Can you work these out from the model? Positions are in its coordinate system, mm. A direction names the side the tool comes from. Round coordinates to 2 decimals unless told otherwise and drop trailing zeros. Order: outer loops, then holes, each group sorted by start corner. A loop starts at its lowest first (then second) coordinate and runs counter-clockwise, first axis right, second up. Notation, with made-up numbers: (27, -17.5) -> (68, -17.5) arc R18 ccw to (68, 7.5) -> close; hole circle Ø4 at (41, -7). An arc over 180 degrees is marked (long way). Use a Markdown table: item, result. Add a question column.
Q1. I need wall thicknesses on line 1 along X through (y, z) = (5.5, 2.85); line 2 along Y through (x, z) = (10, 1.5); line 3 along Y through (x, z) = (-10, 1.6). Which ranges of each line are inside material? Lowest first, please. Write a range as [from, to].
Q2. If we section it at D-D on z = 3.2: Give the number of separate pieces and of enclosed holes in the cut face, plus the area to 3 significant figures.
Q3. If we section it at A-A on x = 0: List the corners of the cut face in (y, z) for me, plus the area to 3 significant figures.
Q4. We'd pull the mould along X, two halves only. Please class faces 1 (the face through (-25.295, -5, 2)), 2 (the face through (0, 45, 2)), 3 (the face through (-27.14, 44.1, 2.03)), 4 (the face through (28, 8, 2)): +X half, -X half, draft (parallel to the pull), parting line (faces both ways), or undercut.
Q5. If we section it at B-B on y = 14.5: List the corners of the cut face in (x, z) for me.
Q6. For faces 5 (the face through (-10.85, 21.08, 2.03)), 6 (the face through (0, 1, 4)), which set-ups out of +Z, -Z, +X, -X, +Y, -Y let a thin tool reach every point of the face, with its end or its side?
Q7. I'm going to push flat-ended pins straight in: pin 1 Ø1.2 at (x, z) = (-18, 1.5) entering from -Y; pin 2 Ø2 at (y, z) = (-27, 3.5) entering from -X (3 decimals); pin 3 Ø2.5 at (x, y) = (-13.44, -3.56) entering from +Z. Where does each tip first touch, or does it pass through?
Q8. If we section it at C-C on y = -16.5: List the corners of the cut face in (x, z) for me, plus the area to 3 significant figures.
```python
from build123d import *

# Parameters (mm, degrees)
SKETCH_1_W          = 56
SKETCH_1_H          = 90
SKETCH_1_R          = 1.6
SKETCH_1_R_2        = 1.3
SKETCH_1_R_3        = 15
EXTRUDE_1_DEPTH     = 4
FILLET_1_R          = 20
CUT_EXTRUDE_1_DEPTH = 54.150729064
FILLET_2_R          = 2
FILLET_3_R          = 3
CUT_EXTRUDE_2_DEPTH = 54.150729064
FILLET_4_R          = 10
FILLET_5_R          = 2
CUT_EXTRUDE_3_DEPTH = 54.150729209
FILLET_6_R          = 1
CUT_EXTRUDE_4_DEPTH = 54.150729209
FILLET_7_R          = 1


with BuildPart() as part:
    # 草图1 → 凸台-拉伸1 (new body)
    with BuildSketch(Plane.XY):
        Rectangle(SKETCH_1_W, SKETCH_1_H)
        with Locations((10, 42)):
            Circle(SKETCH_1_R, mode=Mode.SUBTRACT)
        with Locations(Location((-10, 42, 0), (0, 0, 180))):
            Circle(SKETCH_1_R, mode=Mode.SUBTRACT)
        with Locations((13.435028843, -3.564971157)):
            Circle(SKETCH_1_R_2, mode=Mode.SUBTRACT)
        with Locations((13.435028843, -30.435028843)):
            Circle(SKETCH_1_R_2, mode=Mode.SUBTRACT)
        with Locations((-13.435028843, -30.435028843)):
            Circle(SKETCH_1_R_2, mode=Mode.SUBTRACT)
        with Locations((-13.435028843, -3.564971157)):
            Circle(SKETCH_1_R_2, mode=Mode.SUBTRACT)
        with Locations((0, -17)):
            Circle(SKETCH_1_R_3, mode=Mode.SUBTRACT)
    extrude(amount=EXTRUDE_1_DEPTH)

    # 圆角1
    fillet_1_edges = [part.edges().sort_by_distance(p)[0] for p in [
        (28, -45, 2),
        (-28, -45, 2),
    ]]
    fillet(fillet_1_edges, radius=FILLET_1_R)

    # 草图2 → 切除-拉伸1 (cut, through all)
    with BuildSketch(Plane.XY.offset(4)):
        Polygon((-23.403006558, 36.792468572), (23.403006558, 36.792468572), (0.426117862, 6.963948605), align=None)
        Polygon((-23.403006558, 29.851631864), (-23.403006558, 3.588347177), (-2.422043399, 3.588347177), align=None)
        Polygon((23.403006558, 3.588347177), (2.422043399, 3.588347177), (23.403006558, 29.851631864), align=None)
    extrude(amount=-CUT_EXTRUDE_1_DEPTH, mode=Mode.SUBTRACT)

    # 圆角2
    fillet_2_edges = [part.edges().sort_by_distance(p)[0] for p in [
        (23.403006558, 29.851631864, 2),
        (23.403006558, 3.588347177, 2),
        (2.422043399, 3.588347177, 2),
        (-23.403006558, 29.851631864, 2),
        (-2.422043399, 3.588347177, 2),
        (-23.403006558, 3.588347177, 2),
        (0.426117862, 6.963948605, 2),
        (-23.403006558, 36.792468572, 2),
        (23.403006558, 36.792468572, 2),
    ]]
    fillet(fillet_2_edges, radius=FILLET_2_R)

    # 圆角3
    fillet_3_edges = [part.edges().sort_by_distance(p)[0] for p in [
        (-28, 45, 2),
        (28, 45, 2),
    ]]
    fillet(fillet_3_edges, radius=FILLET_3_R)

    # 草图3 → 切除-拉伸2 (cut, through all)
    with BuildSketch(Plane.XY.offset(4)):
        with BuildLine():
            ThreePointArc((-9.563715622, -28.55574937), (0, -41.141196435), (9.563715622, -28.55574937))
            ThreePointArc((9.563715622, -28.55574937), (0, -32), (-9.563715622, -28.55574937))
        make_face()
        with BuildLine():
            ThreePointArc((-11.55574937, -7.436284378), (-24.141196435, -17), (-11.55574937, -26.563715622))
            ThreePointArc((-11.55574937, -26.563715622), (-15, -17), (-11.55574937, -7.436284378))
        make_face()
        with BuildLine():
            ThreePointArc((11.55574937, -26.563715622), (24.141196435, -17), (11.55574937, -7.436284378))
            ThreePointArc((11.55574937, -7.436284378), (15, -17), (11.55574937, -26.563715622))
        make_face()
    extrude(amount=-CUT_EXTRUDE_2_DEPTH, mode=Mode.SUBTRACT)

    # 圆角4
    fillet_4_edges = [part.edges().sort_by_distance(p)[0] for p in [
        (-11.55574937, -7.436284378, 2),
        (11.55574937, -7.436284378, 2),
    ]]
    fillet(fillet_4_edges, radius=FILLET_4_R)

    # 圆角5
    fillet_5_edges = [part.edges().sort_by_distance(p)[0] for p in [
        (-9.563715622, -28.55574937, 2),
        (9.563715622, -28.55574937, 2),
        (-11.55574937, -26.563715622, 2),
        (11.55574937, -26.563715622, 2),
    ]]
    fillet(fillet_5_edges, radius=FILLET_5_R)

    # 草图4 → 切除-拉伸3 (cut, through all)
    with BuildSketch(Plane.XY.offset(4)):
        Polygon((-22.184991746, -28.213177479), (-10.282808815, -37.433178341), (-7.181535798, -42.46226972), (-17.786358924, -39.94772403), align=None)
        Polygon((7.181535798, -42.46226972), (17.786358924, -39.94772403), (22.184991746, -28.213177479), (10.282808815, -37.433178341), align=None)
    extrude(amount=-CUT_EXTRUDE_3_DEPTH, mode=Mode.SUBTRACT)

    # 圆角6
    fillet_6_edges = [part.edges().sort_by_distance(p)[0] for p in [
        (-17.786358924, -39.94772403, 2),
        (-22.184991746, -28.213177479, 2),
        (-10.282808815, -37.433178341, 2),
        (-7.181535798, -42.46226972, 2),
        (7.181535798, -42.46226972, 2),
        (10.282808815, -37.433178341, 2),
        (22.184991746, -28.213177479, 2),
        (17.786358924, -39.94772403, 2),
    ]]
    fillet(fillet_6_edges, radius=FILLET_6_R)

    # 草图5 → 切除-拉伸4 (cut, through all)
    with BuildSketch(Plane.XY.offset(4)):
        Polygon((-19.572914927, 1.476160836), (-25.295441932, -1.385102666), (-25.295441932, -8.70657104), (-18.394747603, -5.929462346), (-12.756375408, 1.476160836), align=None)
        Polygon((18.394747603, -5.929462346), (12.756375408, 1.476160836), (19.572914927, 1.476160836), (25.295441932, -1.385102666), (25.295441932, -8.70657104), align=None)
    extrude(amount=-CUT_EXTRUDE_4_DEPTH, mode=Mode.SUBTRACT)

    # 圆角7
    fillet_7_edges = [part.edges().sort_by_distance(p)[0] for p in [
        (-19.572914927, 1.476160836, 2),
        (-12.756375408, 1.476160836, 2),
        (-18.394747603, -5.929462346, 2),
        (-25.295441932, -8.70657104, 2),
        (-25.295441932, -1.385102666, 2),
        (25.295441932, -8.70657104, 2),
        (18.394747603, -5.929462346, 2),
        (12.756375408, 1.476160836, 2),
        (19.572914927, 1.476160836, 2),
        (25.295441932, -1.385102666, 2),
    ]]
    fillet(fillet_7_edges, radius=FILLET_7_R)


solid = part.part
```
Answer below:
| question | item | result |
|---|---|---|
| 1 | line 1 | [-28, -23.4], [-4.58, 4.58], [23.4, 28] |
| 1 | line 2 | [-44.9, -41.79], [-37.89, -28.33], [-5.68, 3.59], [13.07, 19.39], [36.79, 40.4], [43.6, 45] |
| 1 | line 3 | [-44.9, -41.79], [-37.89, -28.33], [-5.68, 3.59], [13.07, 20.02], [36.79, 40.4], [43.6, 45] |
| 2 | separate pieces | 1 |
| 2 | enclosed holes | 14 |
| 2 | area | 2,130 mm² |
| 3 | outline | (-45, 0) -> (-41.14, 0) -> (-41.14, 4) -> (-45, 4) -> close; (-2, 0) -> (8.24, 0) -> (8.24, 4) -> (-2, 4) -> close; (36.79, 0) -> (45, 0) -> (45, 4) -> (36.79, 4) -> close |
| 3 | area | 89.2 mm² |
| 4 | face 1 | undercut |
| 4 | face 2 | draft |
| 4 | face 3 | -X half |
| 4 | face 4 | +X half |
| 5 | outline | (-28, 0) -> (-23.4, 0) -> (-23.4, 4) -> (-28, 4) -> close; (-11.14, 0) -> (-5.59, 0) -> (-5.59, 4) -> (-11.14, 4) -> close; (6.23, 0) -> (11.14, 0) -> (11.14, 4) -> (6.23, 4) -> close; (23.4, 0) -> (28, 0) -> (28, 4) -> (23.4, 4) -> close |
| 6 | face 5 | +Z, -Z |
| 6 | face 6 | +Z, +X, -X, +Y, -Y |
| 7 | pin 1 | y = -42.65 |
| 7 | pin 2 | x = -27.975 |
| 7 | pin 3 | through |
| 8 | outline | (-28, 0) -> (-24.13, 0) -> (-24.13, 4) -> (-28, 4) -> close; (24.13, 0) -> (28, 0) -> (28, 4) -> (24.13, 4) -> close |
| 8 | area | 31.0 mm² |
